Part model, mm, in its own coordinate system. A direction names the side the tool comes from. Round coordinates to 2 decimals unless told otherwise and drop trailing zeros. Loops run counter-clockwise (first coordinate to the right, second up) from the corner with the lowest first, then second, coordinate; pieces in that order, holes last.
(1) Cut at B-B on y = 27. List the corners of the cut face in (x, z).
(2) Cut at A-A on z = 0.7. List the corners of the cut face in (x, y).
(3) Flat gauge pins, fed straight in: pin 1 (2 mm diameter, centred on y = 5, z = 2.5, fed in from +X); pin 2 (1.5 mm diameter, centred on y = 4, z = 3, fed in from +X); pin 3 (1.2 mm diameter, centred on y = 22, z = 2, fed in from -X). Where does each tip first touch, or does it go through?
(4) Tool access for faces 1 (the face through (2.12, 3.74, 1.97)), 2 (the face through (4.65, 23, 2)), 3 (the face through (-4.65, 23, 2)): list every direction of +Z, -Z, +X, -X, +Y, -Y with a clear straight run to the whole face (end or side of a thin tool).
(5) Cut at C-C on x = -6.8. List the corners of the cut face in (y, z), then the cut area to 3 significant figures.
(6) Probe probe 1 along Y at (x, z) = (0, 2.65); probe 2 along X at (y, z) = (4.5, 2.85); probe 3 along X at (y, z) = (11.5, 1.65). List the from-to ranges inside material, lowest first.
(7) Mould opens along X. For faces 4 (the face through (-4.3, 0, 2)), 5 (the face through (-0.434, 35.328, 2.028)), 6 (the face through (0, 19, 4)), 7 (the face through (8.91, 4.34, 2.03)) say: +X half, -X half, draft (parallel to the pull), parting line (faces both ways), or undercut.
from build123d import *

# Parameters (mm, degrees)
F1_DEPTH = 4
F2_R     = 3
F3_R     = 2
F4_DEPTH = 4


with BuildPart() as f1:
    # F0 (on Top) → F1 (new body)
    with BuildSketch(Plane.XY):
        Polygon((-4.3, 2.482606), (0, 4.965212), (0, 9.965212), (-4.65, 7.280534), (-9.3, 4.595855), (-9.3, -2.482606), (-4.3, -2.482606), align=None)
        Polygon((0, 4.965212), (4.3, 2.482606), (4.3, -2.482606), (9.3, -2.482606), (9.3, 4.595855), (4.65, 7.280534), (0, 9.965212), align=None)
        with BuildLine():
            Line((-4.65, 7.280534), (0, 9.965212))
            Line((0, 9.965212), (4.65, 7.280534))
            Line((4.65, 7.280534), (4.65, 37.280534))
            ThreePointArc((4.65, 37.280534), (0, 41.930534), (-4.65, 37.280534))
            Line((-4.65, 37.280534), (-4.65, 7.280534))
        make_face()
        with BuildLine():
            ThreePointArc((-9.3, -2.482606), (-6.8, -4.982606), (-4.3, -2.482606))
            Line((-4.3, -2.482606), (-9.3, -2.482606))
        make_face()
        with BuildLine():
            Line((9.3, -2.482606), (4.3, -2.482606))
            ThreePointArc((4.3, -2.482606), (6.8, -4.982606), (9.3, -2.482606))
        make_face()
    extrude(amount=F1_DEPTH)

    # F2
    f2_edges = [f1.edges().sort_by_distance(p)[0] for p in [
        (9.3, 4.595855, 2),
        (4.65, 7.280534, 2),
        (-4.65, 7.280534, 2),
        (-9.3, 4.595855, 2),
    ]]
    fillet(f2_edges, radius=F2_R)

    # F3 (on face) → F4 (cut, through all)
    with BuildSketch(Plane.XY.offset(4)):
        with Locations((0, 37.280534)):
            Circle(F3_R)
    extrude(amount=-F4_DEPTH, mode=Mode.SUBTRACT)


solid = f1.part
Final values:
1. outline: (-4.65, 0) - (4.65, 0) - (4.65, 4) - (-4.65, 4) - close
2. outline: (-9.3, -2.48) arc R2.5 ccw to (-4.3, -2.48) - (-4.3, 2.48) - (0, 4.97) - (4.3, 2.48) - (4.3, -2.48) arc R2.5 ccw to (9.3, -2.48) - (9.3, 2.86) arc R3 ccw to (7.8, 5.46) - (6.15, 6.41) arc R3 cw to (4.65, 9.01) - (4.65, 37.28) arc R4.65 ccw to (-4.65, 37.28) - (-4.65, 9.01) arc R3 cw to (-6.15, 6.41) - (-7.8, 5.46) arc R3 ccw to (-9.3, 2.86) - close; hole circle Ø4 at (0, 37.28)
3. pin 1: stops at x = 9.08
3. pin 2: stops at x = 9.28
3. pin 3: stops at x = -4.65
4. face 1: +Z, -Z, -Y
4. face 2: +Z, -Z, +X, +Y
4. face 3: +Z, -Z, -X, +Y
5. outline: (-4.98, 0) - (6.04, 0) - (6.04, 4) - (-4.98, 4) - close
5. area: 44.1 mm2
6. probe 1: y = 4.97 to 35.28, 39.28 to 41.93
6. probe 2: x = -8.81 to -0.81, 0.81 to 8.81
6. probe 3: x = -4.65 to 4.65
7. face 4: undercut
7. face 5: undercut
7. face 6: draft
7. face 7: +X half
